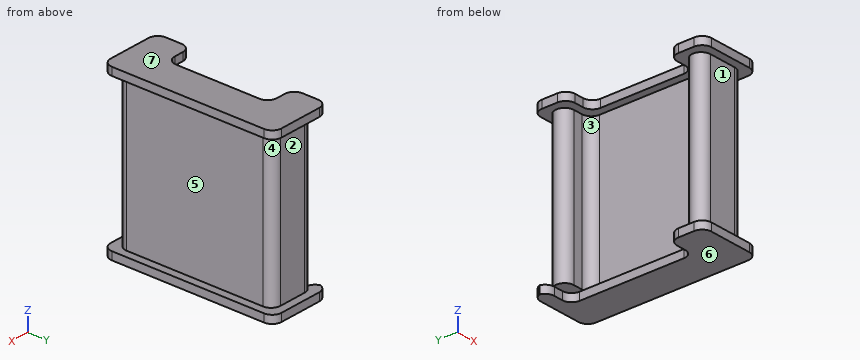
from build123d import *

# Parameters (mm, degrees)
BOSS_EXTRUDE1_DEPTH = 48.42
BOSS_EXTRUDE2_DEPTH = 2.54
BOSS_EXTRUDE3_DEPTH = 2.54
FILLET4_R           = 3
FILLET5_R           = 3


with BuildPart() as part:
    # Sketch1 → Boss-Extrude1 (new body)
    with BuildSketch(Plane.XY):
        Polygon((0, 6), (0, 0), (15, 0), (15, 46.604118993), (15, 50), (0, 50), (0, 44), (9, 44), (9, 6), align=None)
    extrude(amount=BOSS_EXTRUDE1_DEPTH)

    # Sketch2 → Boss-Extrude2 (add)
    with BuildSketch(Plane.XY.offset(48.42)):
        Polygon((-2.54, 41.46), (6.46, 41.46), (6.46, 8.54), (-2.54, 8.54), (-2.54, -2.54), (17.54, -2.54), (17.54, 52.54), (-2.54, 52.54), align=None)
    extrude(amount=BOSS_EXTRUDE2_DEPTH)

    # Sketch3 → Boss-Extrude3 (add)
    with BuildSketch(Plane(origin=(0, 0, 0), x_dir=(-1, 0, 0), z_dir=(0, 0, -1))):
        Polygon((2.54, 52.54), (-17.54, 52.54), (-17.54, 48.156890446), (-17.54, -2.54), (-6.46, -2.54), (2.54, -2.54), (2.54, 8.54), (-6.46, 8.54), (-6.46, 48.156890446), (2.54, 48.156890446), align=None)
    extrude(amount=BOSS_EXTRUDE3_DEPTH)

    # Fillet4
    # the kernel refuses this fillet: 3 mm, written as the material it adds along each edge
    with BuildSketch(Plane(origin=(9, 6, -7.5), x_dir=(0, 1, 0), z_dir=(0, 0, 1))) as fillet4_piece_1_section:
        with BuildLine():
            CenterArc((FILLET4_R, FILLET4_R), FILLET4_R, 180, 90)
            Line((0, FILLET4_R), (0, 0))
            Line((0, 0), (FILLET4_R, 0))
        make_face()
    fillet4_piece_1 = extrude(amount=63.42, mode=Mode.PRIVATE)
    fillet4_piece_1 = split(fillet4_piece_1, bisect_by=Plane(origin=(8.329896183, 6.670103817, 50.96), z_dir=(0, 0, -1)), keep=Keep.TOP, mode=Mode.PRIVATE)
    fillet4_piece_1 = split(fillet4_piece_1, bisect_by=Plane(origin=(8.329896183, 6.670103817, -2.54), z_dir=(0, 0, 1)), keep=Keep.TOP, mode=Mode.PRIVATE)
    add(fillet4_piece_1)
    with BuildSketch(Plane(origin=(9, 44, 0), x_dir=(-1, 0, 0), z_dir=(0, 0, 1))) as fillet4_piece_2_section:
        with BuildLine():
            CenterArc((FILLET4_R, FILLET4_R), FILLET4_R, 180, 90)
            Line((0, FILLET4_R), (0, 0))
            Line((0, 0), (FILLET4_R, 0))
        make_face()
    fillet4_piece_2 = extrude(amount=55.92, mode=Mode.PRIVATE)
    fillet4_piece_2 = split(fillet4_piece_2, bisect_by=Plane(origin=(6.34513643, 43.989367947, 50.96), z_dir=(0, 0, -1)), keep=Keep.TOP, mode=Mode.PRIVATE)
    add(fillet4_piece_2)
    # the kernel refuses this fillet: 3 mm, written as the material it takes off along each edge
    with BuildSketch(Plane(origin=(0, 6, 0), x_dir=(0, -1, 0), z_dir=(0, 0, 1)), Plane(origin=(15, 0, 0), x_dir=(0, 1, 0), z_dir=(0, 0, 1)), Plane(origin=(0, 0, 0), x_dir=(1, 0, 0), z_dir=(0, 0, 1)), Plane(origin=(0, 50, 0), x_dir=(0, -1, 0), z_dir=(0, 0, 1))) as fillet4_2_piece_1:
        with BuildLine():
            CenterArc((FILLET4_R, FILLET4_R), FILLET4_R, 180, 90)
            Line((0, FILLET4_R), (0, 0))
            Line((0, 0), (FILLET4_R, 0))
        make_face()
    extrude(amount=48.42, mode=Mode.SUBTRACT)
    with BuildSketch(Plane(origin=(15, 50, 0), x_dir=(0, -1, 0), z_dir=(0, 0, 1))) as fillet4_2_piece_2:
        with BuildLine():
            CenterArc((FILLET4_R, -FILLET4_R), FILLET4_R, 90, 90)
            Line((0, -FILLET4_R), (0, 0))
            Line((0, 0), (FILLET4_R, 0))
        make_face()
    extrude(amount=48.42, mode=Mode.SUBTRACT)
    with BuildSketch(Plane(origin=(0, 44, -7.5), x_dir=(1, 0, 0), z_dir=(0, 0, 1))) as fillet4_2_piece_3:
        with BuildLine():
            CenterArc((FILLET4_R, FILLET4_R), FILLET4_R, 180, 90)
            Line((0, FILLET4_R), (0, 0))
            Line((0, 0), (FILLET4_R, 0))
        make_face()
    extrude(amount=55.92, mode=Mode.SUBTRACT)

    # Fillet5
    # the kernel refuses this fillet: 3 mm, written as the material it adds along each edge
    with BuildSketch(Plane(origin=(6.46, 41.46, 48.42), x_dir=(0, -1, 0), z_dir=(0, 0, 1)), Plane(origin=(6.46, 8.54, 48.42), x_dir=(-1, 0, 0), z_dir=(0, 0, 1)), Plane(origin=(6.46, 8.54, 0), x_dir=(0, 1, 0), z_dir=(0, 0, -1))) as fillet5_piece_1:
        with BuildLine():
            CenterArc((FILLET5_R, -FILLET5_R), FILLET5_R, 90, 90)
            Line((0, -FILLET5_R), (0, 0))
            Line((0, 0), (FILLET5_R, 0))
        make_face()
    extrude(amount=2.54)
    with BuildSketch(Plane(origin=(6.46, 48.156890446, 7.5), x_dir=(0, -1, 0), z_dir=(0, 0, -1))) as fillet5_piece_2:
        with BuildLine():
            CenterArc((FILLET5_R, FILLET5_R), FILLET5_R, 180, 90)
            Line((0, FILLET5_R), (0, 0))
            Line((0, 0), (FILLET5_R, 0))
        make_face()
    extrude(amount=10.04)
    # the kernel refuses this fillet: 3 mm, written as the material it takes off along each edge
    with BuildSketch(Plane(origin=(-2.54, 52.54, 40.92), x_dir=(1, 0, 0), z_dir=(0, 0, 1)), Plane(origin=(-2.54, 8.54, 40.92), x_dir=(1, 0, 0), z_dir=(0, 0, 1)), Plane(origin=(-2.54, -2.54, 40.92), x_dir=(0, 1, 0), z_dir=(0, 0, 1)), Plane(origin=(17.54, -2.54, 40.92), x_dir=(-1, 0, 0), z_dir=(0, 0, 1)), Plane(origin=(17.54, 52.54, 40.92), x_dir=(0, -1, 0), z_dir=(0, 0, 1)), Plane(origin=(-2.54, 52.54, 7.5), x_dir=(0, -1, 0), z_dir=(0, 0, -1)), Plane(origin=(17.54, 52.54, 7.5), x_dir=(-1, 0, 0), z_dir=(0, 0, -1)), Plane(origin=(17.54, -2.54, 7.5), x_dir=(0, 1, 0), z_dir=(0, 0, -1)), Plane(origin=(-2.54, -2.54, 7.5), x_dir=(1, 0, 0), z_dir=(0, 0, -1)), Plane(origin=(-2.54, 8.54, 7.5), x_dir=(0, -1, 0), z_dir=(0, 0, -1))) as fillet5_2_piece_1:
        with BuildLine():
            CenterArc((FILLET5_R, -FILLET5_R), FILLET5_R, 90, 90)
            Line((0, -FILLET5_R), (0, 0))
            Line((0, 0), (FILLET5_R, 0))
        make_face()
    extrude(amount=17.54, mode=Mode.SUBTRACT)
    with BuildSketch(Plane(origin=(-2.54, 41.46, 40.92), x_dir=(1, 0, 0), z_dir=(0, 0, 1))) as fillet5_2_piece_2:
        with BuildLine():
            CenterArc((FILLET5_R, FILLET5_R), FILLET5_R, 180, 90)
            Line((0, FILLET5_R), (0, 0))
            Line((0, 0), (FILLET5_R, 0))
        make_face()
    extrude(amount=17.54, mode=Mode.SUBTRACT)
    with BuildSketch(Plane(origin=(-2.54, 48.156890446, 0), x_dir=(1, 0, 0), z_dir=(0, 0, -1))) as fillet5_2_piece_3:
        with BuildLine():
            CenterArc((FILLET5_R, -FILLET5_R), FILLET5_R, 90, 90)
            Line((0, -FILLET5_R), (0, 0))
            Line((0, 0), (FILLET5_R, 0))
        make_face()
    extrude(amount=10.04, mode=Mode.SUBTRACT)


solid = part.part
Can you work these out from the model? Positions are in its coordinate system, mm. Face numbers are marked on the shaded views. A direction names the side the tool comes from. Give positions to 0.01 mm unless a question says otherwise; leave off trailing zeros. Loops run counter-clockwise (first coordinate to the right, second up) from the corner with the lowest first, then second, coordinate; pieces in that order, holes last. Notation, with made-up numbers: (23.25, 56) - (38.25, 56) arc R25 cw to (38.25, 94) - close; hole circle Ø2 at (78.5, -11.5). An arc over 180 degrees is marked (long way). Answer as a JSON object with one key per item and string values.
Q1. If I drill on L1, parallel to Y at x = 5.25, z = 47; L2, parallel to Z at x = 8.25, y = 22.5; L3, parallel to Y at x = 12, z = 14.5, over which ranges is the centre line in solid material (lowest first)?
Geometry says:
{"L1": "0 to 6, 44 to 50", "L2": "-2.54 to 0, 48.42 to 50.96", "L3": "0 to 50"}
Q2. Imagine slicing it at B-B on y = 28. Write out the boundary of the cut face in (x, z), plus the area to 3 significant figures.
Geometry says:
{"outline": "(6.46, -2.54) - (17.54, -2.54) - (17.54, 0) - (15, 0) - (15, 48.42) - (17.54, 48.42) - (17.54, 50.96) - (6.46, 50.96) - (6.46, 48.42) - (9, 48.42) - (9, 0) - (6.46, 0) - close", "area": "347 mm²"}
Q3. Will these pins go through, and if not, where does the flat tip stop? P1, Ø10, axis at y = 35, z = 16.5, coming from the -X side; P2, Ø3.5, axis at x = 5, z = 24.5, coming from the -Y side; P3, Ø2, axis at x = 3.5, y = 47, coming from the -Z side.
Geometry says:
{"P1": "x = 9", "P2": "y = 0", "P3": "z = 0"}
Q4. Which directions (+Z, -Z, +X, -X, +Y, -Y) give clear straight access to the entire face, cutting with the end or side of a thin tool? Please do the marked faces 1, 2 and 3.
Geometry says:
{"face 1": "+X, -X, -Y", "face 2": "+X, -X, +Y", "face 3": "-X"}
Q5. If we mould it in two halves opening along Z, with no side actions, what happens to the marked faces 4, 5, 6 and 7? For each: pulls with the +Z half, pulls with the -Z half, needs draft (parallel to the pull), parting line crosses it, or undercut.
Geometry says:
{"face 4": "undercut", "face 5": "undercut", "face 6": "pulls with the -Z half", "face 7": "pulls with the +Z half"}
Q6. Imagine slicing it at A-A on z = 36.5. Write out the boundary of the cut face in (x, y).
Geometry says:
{"outline": "(3, 0) - (12, 0) arc R3 ccw to (15, 3) - (15, 47) arc R3 ccw to (12, 50) - (3, 50) arc R3 ccw to (3, 44) - (6, 44) arc R3 cw to (9, 41) - (9, 9) arc R3 cw to (6, 6) - (3, 6) arc R3 ccw to start"}
Q7. Imagine slicing it at C-C on x = 7.25. Write out the boundary of the cut face in (y, z), plus the area to 3 significant figures.
Geometry says:
{"outline": "(-2.54, -2.54) - (52.54, -2.54) - (52.54, 0) - (50, 0) - (50, 48.42) - (52.54, 48.42) - (52.54, 50.96) - (-2.54, 50.96) - (-2.54, 48.42) - (0, 48.42) - (0, 0) - (-2.54, 0) - close; hole (6.27, 0) - (43.73, 0) - (43.73, 48.42) - (6.27, 48.42) - close", "area": "887 mm²"}
